from build123d import *

# Parameters (mm, degrees)
SKETCH1_W           = 3
SKETCH1_H           = 3
SKETCH1_W_2         = 3.744317383
SKETCH1_H_2         = 3.744317383
BOSS_EXTRUDE1_DEPTH = 3


with BuildPart() as part:
    # Sketch1 → Boss-Extrude1 (new body)
    with BuildSketch(Plane.XY):
        Polygon((12, 297), (3, 288), (3, 174), (12, 165), (126, 165), (135, 174), (135, 288), (126, 297), align=None)
        with Locations((57, 285)):
            Rectangle(SKETCH1_W, SKETCH1_H, mode=Mode.SUBTRACT)
        with Locations((81, 285)):
            Rectangle(SKETCH1_W, SKETCH1_H, mode=Mode.SUBTRACT)
        with Locations((21, 285)):
            Rectangle(SKETCH1_W, SKETCH1_H, mode=Mode.SUBTRACT)
        with Locations((117, 285)):
            Rectangle(SKETCH1_W, SKETCH1_H, mode=Mode.SUBTRACT)
        with Locations((81, 177)):
            Rectangle(SKETCH1_W, SKETCH1_H, mode=Mode.SUBTRACT)
        with Locations((57, 177)):
            Rectangle(SKETCH1_W, SKETCH1_H, mode=Mode.SUBTRACT)
        with Locations((117, 177)):
            Rectangle(SKETCH1_W, SKETCH1_H, mode=Mode.SUBTRACT)
        with Locations((21, 177)):
            Rectangle(SKETCH1_W, SKETCH1_H, mode=Mode.SUBTRACT)
        with Locations((15, 279)):
            Rectangle(SKETCH1_W, SKETCH1_H, mode=Mode.SUBTRACT)
        with Locations((15, 183)):
            Rectangle(SKETCH1_W, SKETCH1_H, mode=Mode.SUBTRACT)
        with Locations((15, 243)):
            Rectangle(SKETCH1_W, SKETCH1_H, mode=Mode.SUBTRACT)
        with Locations((15, 219)):
            Rectangle(SKETCH1_W, SKETCH1_H, mode=Mode.SUBTRACT)
        with Locations((123, 183)):
            Rectangle(SKETCH1_W, SKETCH1_H, mode=Mode.SUBTRACT)
        with Locations((123, 279)):
            Rectangle(SKETCH1_W, SKETCH1_H, mode=Mode.SUBTRACT)
        with Locations((123, 219)):
            Rectangle(SKETCH1_W, SKETCH1_H, mode=Mode.SUBTRACT)
        with Locations((123, 243)):
            Rectangle(SKETCH1_W, SKETCH1_H, mode=Mode.SUBTRACT)
        with Locations((17.66659907, 212.625)):
            Rectangle(SKETCH1_W_2, SKETCH1_H, mode=Mode.SUBTRACT)
        with Locations((17.66659907, 254.625)):
            Rectangle(SKETCH1_W_2, SKETCH1_H, mode=Mode.SUBTRACT)
        with Locations((17.66659907, 233.625)):
            Rectangle(SKETCH1_W_2, SKETCH1_H, mode=Mode.SUBTRACT)
        with Locations((17.66659907, 275.625)):
            Rectangle(SKETCH1_W_2, SKETCH1_H, mode=Mode.SUBTRACT)
        with Locations((17.66659907, 191.625)):
            Rectangle(SKETCH1_W_2, SKETCH1_H, mode=Mode.SUBTRACT)
        with Locations((87.375, 179.666599071)):
            Rectangle(SKETCH1_W, SKETCH1_H_2, mode=Mode.SUBTRACT)
        with Locations((45.375, 179.666599071)):
            Rectangle(SKETCH1_W, SKETCH1_H_2, mode=Mode.SUBTRACT)
        with Locations((66.375, 179.666599071)):
            Rectangle(SKETCH1_W, SKETCH1_H_2, mode=Mode.SUBTRACT)
        with Locations((24.375, 179.666599071)):
            Rectangle(SKETCH1_W, SKETCH1_H_2, mode=Mode.SUBTRACT)
        with Locations((108.375, 179.666599071)):
            Rectangle(SKETCH1_W, SKETCH1_H_2, mode=Mode.SUBTRACT)
        with Locations((120.33340093, 249.375)):
            Rectangle(SKETCH1_W_2, SKETCH1_H, mode=Mode.SUBTRACT)
        with Locations((120.33340093, 207.375)):
            Rectangle(SKETCH1_W_2, SKETCH1_H, mode=Mode.SUBTRACT)
        with Locations((120.33340093, 228.375)):
            Rectangle(SKETCH1_W_2, SKETCH1_H, mode=Mode.SUBTRACT)
        with Locations((120.33340093, 186.375)):
            Rectangle(SKETCH1_W_2, SKETCH1_H, mode=Mode.SUBTRACT)
        with Locations((120.33340093, 270.375)):
            Rectangle(SKETCH1_W_2, SKETCH1_H, mode=Mode.SUBTRACT)
        with Locations((50.625, 282.33340093)):
            Rectangle(SKETCH1_W, SKETCH1_H_2, mode=Mode.SUBTRACT)
        with Locations((92.625, 282.33340093)):
            Rectangle(SKETCH1_W, SKETCH1_H_2, mode=Mode.SUBTRACT)
        with Locations((71.625, 282.33340093)):
            Rectangle(SKETCH1_W, SKETCH1_H_2, mode=Mode.SUBTRACT)
        with Locations((113.625, 282.33340093)):
            Rectangle(SKETCH1_W, SKETCH1_H_2, mode=Mode.SUBTRACT)
        with Locations((29.625, 282.33340093)):
            Rectangle(SKETCH1_W, SKETCH1_H_2, mode=Mode.SUBTRACT)
    extrude(amount=BOSS_EXTRUDE1_DEPTH)


solid = part.part
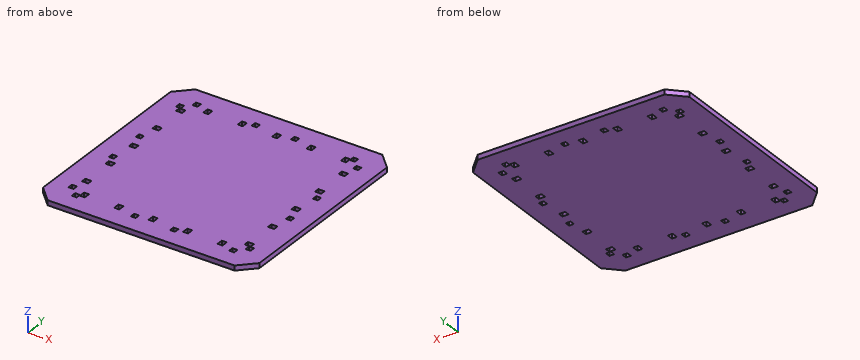
Can you work these out from the model? Positions are in its coordinate system, mm. Give positions to 0.01 mm unless a question says otherwise; leave off trailing zeros. Order: outer loops, then holes, each group sorted by start corner. A loop starts at its lowest first (then second) coordinate and runs counter-clockwise, first axis right, second up. Notation, with made-up numbers: (-1, 39.25) - (18, 39.25) arc R7 ccw to (18, 49.25) - close; hole circle Ø8 at (63.5, 16). An arc over 180 degrees is marked (long way). Write each question's results on one line, items separated by ' | '.
1) Please list where these lines run through material, in increasing order: line 1 along X through (y, z) = (220, 1.15); line 2 along X through (y, z) = (177, 1.65); line 3 along X through (y, z) = (255.5, 0.95). Write a range as [from, to].
Final values:
line 1: x = [3, 13.5], [16.5, 121.5], [124.5, 135] | line 2: x = [3, 19.5], [22.5, 55.5], [58.5, 79.5], [82.5, 115.5], [118.5, 135] | line 3: x = [3, 15.79], [19.54, 135]
2) Suppose I cut it at A-A, the plane y = 180. Write out the boundary of the cut face in (x, z) (3 decimals).
Final values:
outline: (3, 0) - (22.875, 0) - (22.875, 3) - (3, 3) - close; (25.875, 0) - (43.875, 0) - (43.875, 3) - (25.875, 3) - close; (46.875, 0) - (64.875, 0) - (64.875, 3) - (46.875, 3) - close; (67.875, 0) - (85.875, 0) - (85.875, 3) - (67.875, 3) - close; (88.875, 0) - (106.875, 0) - (106.875, 3) - (88.875, 3) - close; (109.875, 0) - (135, 0) - (135, 3) - (109.875, 3) - close
3) I'm going to push a flat-ended pin straight in: pin 1 Ø5 at (x, y) = (44.5, 263) entering from -Z. Where does the tip first touch, or does it pass through?
Final values:
pin 1: stops at z = 0
4) Suppose I cut it at B-B, the plane z = 0.9. Give the number of separate pieces and of enclosed holes in the cut face, then the cut area to 3 significant figures.
Final values:
separate pieces: 1 | enclosed holes: 36 | area: 16,900 mm^2
